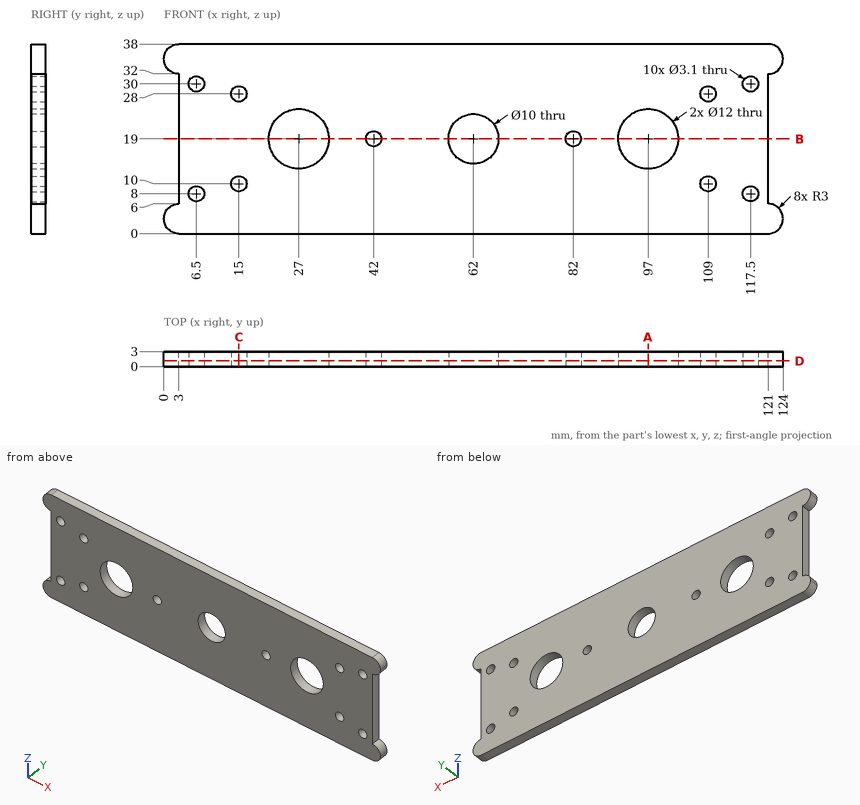
Could you check a few things on this drawing? It's one solid part, dimensions in mm from its lowest x, y, z. Coordinates: 2 decimals unless noted, no trailing zeros. Order: outer loops, then holes, each group sorted by start corner. A loop starts at its lowest first (then second) coordinate and runs counter-clockwise, first axis right, second up. Notation, with made-up numbers: (-24.5, 63.5) - (11.5, 63.5) arc R19 ccw to (11.5, 96.5) - close; hole circle Ø3 at (29, 33.25). An arc over 180 degrees is marked (long way). One line per question, with ' | ' between items.
(1) Suppose I cut it at A-A on x = 97. List the corners of the cut face in (y, z) for me.
Report:
outline: (0, 0) - (3, 0) - (3, 13) - (0, 13) - close; (0, 25) - (3, 25) - (3, 38) - (0, 38) - close
(2) Suppose I cut it at C-C on x = 15. List the corners of the cut face in (y, z) for me, and give its area (3 significant figures).
Report:
outline: (0, 0) - (3, 0) - (3, 8.45) - (0, 8.45) - close; (0, 11.55) - (3, 11.55) - (3, 26.45) - (0, 26.45) - close; (0, 29.55) - (3, 29.55) - (3, 38) - (0, 38) - close | area: 95.4 mm2
(3) Suppose I cut it at B-B on z = 19. List the corners of the cut face in (x, y) for me, and give its area (3 significant figures).
Report:
outline: (3, 0) - (21, 0) - (21, 3) - (3, 3) - close; (33, 0) - (40.45, 0) - (40.45, 3) - (33, 3) - close; (43.55, 0) - (57, 0) - (57, 3) - (43.55, 3) - close; (67, 0) - (80.45, 0) - (80.45, 3) - (67, 3) - close; (83.55, 0) - (91, 0) - (91, 3) - (83.55, 3) - close; (103, 0) - (121, 0) - (121, 3) - (103, 3) - close | area: 233 mm2
(4) If I drill on L1, parallel to X at y = 1.25, z = 28; L2, parallel to Z at x = 15, y = 2.1; L3, parallel to X at y = 1.9, z = 19, over which ranges is the centre line in solid material (lowest first)?
Report:
L1: x = 3 to 13.45, 16.55 to 107.45, 110.55 to 121 | L2: z = 0 to 8.45, 11.55 to 26.45, 29.55 to 38 | L3: x = 3 to 21, 33 to 40.45, 43.55 to 57, 67 to 80.45, 83.55 to 91, 103 to 121
(5) Suppose I cut it at D-D on y = 1.15. State how many separate pieces and enclosed holes the cut face has, and give its area (3 significant figures).
Report:
separate pieces: 1 | enclosed holes: 13 | area: 4,160 mm2
